from build123d import *

# Parameters (mm, degrees)
BOSS_EXTRUDE1_DEPTH        = 7.7
F_6_7_6_7_DIAMETER_HOLE1_D = 6.7
F_8_0_8_DIAMETER_HOLE1_D   = 8


with BuildPart() as part:
    # Sketch1 → Boss-Extrude1 (new body)
    with BuildSketch(Plane.XY):
        with BuildLine():
            Line((-40, 25), (40, 25))
            Line((40, 25), (40, 5.5))
            Line((40, 5.5), (18.5, 5.5))
            ThreePointArc((18.5, 5.5), (13, 0), (18.5, -5.5))
            Line((18.5, -5.5), (40, -5.5))
            Line((40, -5.5), (40, -25))
            Line((40, -25), (-40, -25))
            Line((-40, -25), (-40, -5.5))
            Line((-40, -5.5), (-18.5, -5.5))
            ThreePointArc((-18.5, -5.5), (-13, 0), (-18.5, 5.5))
            Line((-18.5, 5.5), (-40, 5.5))
            Line((-40, 5.5), (-40, 25))
        make_face()
    extrude(amount=BOSS_EXTRUDE1_DEPTH)

    # Ø6.7 (6.7) Diameter Hole1 (through all)
    with Locations(Plane.XY.offset(7.7)):
        with Locations((31, 18), (-31, 18), (-31, -18), (31, -18)):
            Hole(F_6_7_6_7_DIAMETER_HOLE1_D / 2)

    # Ø8.0 (8) Diameter Hole1 (through all)
    with Locations(Plane.XY.offset(7.7)):
        with Locations((0, 0)):
            Hole(F_8_0_8_DIAMETER_HOLE1_D / 2)


solid = part.part
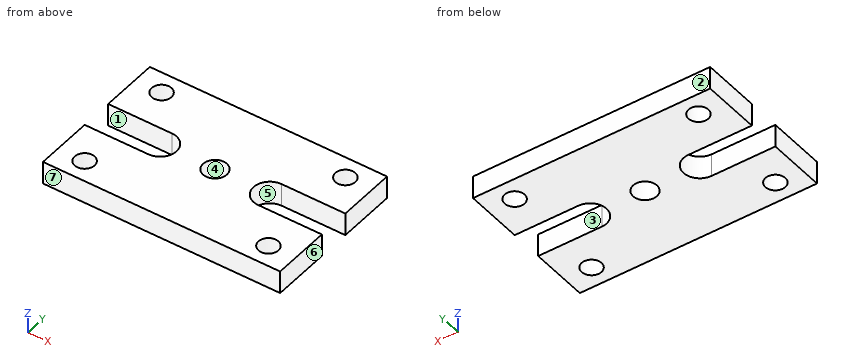
Could you check a few things on this model? Use its own coordinates, in mm. Face numbers are marked on the shaded views. A direction names the side the tool comes from. Give positions to 0.01 mm unless a question says otherwise; leave off trailing zeros. Write each loop counter-clockwise with the first axis right and the second up, starting at its lowest first coordinate (ties: lowest second). Pieces come first, ordered by that corner, then holes. Notation, with made-up numbers: (37, -22.75) -> (67, -22.75) arc R19 cw to (67, 6.25) -> close; hole circle Ø6 at (-5.75, -32.5). An arc over 180 degrees is marked (long way). Answer as a JSON object with one key per item and string values.
Q1. We'd pull the mould along Y, two halves only. Please class the marked faces 4, 5, 6 and 7: released by +Y, released by -Y, zero draft, split by the parting line, or undercut.
Taken from the geometry:
{"face 4": "undercut", "face 5": "undercut", "face 6": "zero draft", "face 7": "released by -Y"}
Q2. Suppose I cut it at B-B on x = -23. Write out the boundary of the cut face in (y, z), then the cut area to 3 significant figures.
Taken from the geometry:
{"outline": "(-25, 0) -> (-5.5, 0) -> (-5.5, 7.7) -> (-25, 7.7) -> close; (5.5, 0) -> (25, 0) -> (25, 7.7) -> (5.5, 7.7) -> close", "area": "300 mm²"}
Q3. Suppose I cut it at C-C on z = 5. Write out the boundary of the cut face in (x, y).
Taken from the geometry:
{"outline": "(-40, -25) -> (40, -25) -> (40, -5.5) -> (18.5, -5.5) arc R5.5 cw to (18.5, 5.5) -> (40, 5.5) -> (40, 25) -> (-40, 25) -> (-40, 5.5) -> (-18.5, 5.5) arc R5.5 cw to (-18.5, -5.5) -> (-40, -5.5) -> close; hole circle Ø6.7 at (-31, -18); hole circle Ø6.7 at (-31, 18); hole circle Ø8 at (0, 0); hole circle Ø6.7 at (31, -18); hole circle Ø6.7 at (31, 18)"}
Q4. Suppose I cut it at A-A on y = -18. Write out the boundary of the cut face in (x, z).
Taken from the geometry:
{"outline": "(-40, 0) -> (-34.35, 0) -> (-34.35, 7.7) -> (-40, 7.7) -> close; (-27.65, 0) -> (27.65, 0) -> (27.65, 7.7) -> (-27.65, 7.7) -> close; (34.35, 0) -> (40, 0) -> (40, 7.7) -> (34.35, 7.7) -> close"}
Q5. Which directions (+Z, -Z, +X, -X, +Y, -Y) give clear straight access to the entire face, cutting with the end or side of a thin tool? Please do the marked faces 1, 2 and 3.
Taken from the geometry:
{"face 1": "+Z, -Z, -X", "face 2": "+Z, -Z, +X, -X, +Y", "face 3": "+Z, -Z, +X"}
Q6. Please list where these lines run through material, in increasing order: L1, parallel to Y at x = 31, z = 6.25; L2, parallel to Y at x = 25.5, z = 2.5; L3, parallel to Y at x = 30, z = 6.
Taken from the geometry:
{"L1": "y = -25 to -21.35, -14.65 to -5.5, 5.5 to 14.65, 21.35 to 25", "L2": "y = -25 to -5.5, 5.5 to 25", "L3": "y = -25 to -21.2, -14.8 to -5.5, 5.5 to 14.8, 21.2 to 25"}
Q7. Suppose I cut it at D-D on x = 31. Write out the boundary of the cut face in (y, z), then the cut area to 3 significant figures.
Taken from the geometry:
{"outline": "(-25, 0) -> (-21.35, 0) -> (-21.35, 7.7) -> (-25, 7.7) -> close; (-14.65, 0) -> (-5.5, 0) -> (-5.5, 7.7) -> (-14.65, 7.7) -> close; (5.5, 0) -> (14.65, 0) -> (14.65, 7.7) -> (5.5, 7.7) -> close; (21.35, 0) -> (25, 0) -> (25, 7.7) -> (21.35, 7.7) -> close", "area": "197 mm²"}
